from build123d import *
from OCP.BRepFilletAPI import BRepFilletAPI_MakeChamfer

# Parameters (mm, degrees)
BOSS_EXTRUDE1_START = -0.635
SKETCH3_R           = 9.525
SKETCH3_R_2         = 4.9657
BOSS_EXTRUDE1_DEPTH = 1.27
CHAMFER1_SIZE       = 0.127
CHAMFER1_SIZE2      = 0.073323484
FILLET1_R           = 0.381


with BuildPart() as part:
    # Sketch3 → Boss-Extrude1 (new body)
    with BuildSketch(Plane.XY.offset(BOSS_EXTRUDE1_START)):
        Circle(SKETCH3_R)
        Circle(SKETCH3_R_2, mode=Mode.SUBTRACT)
    extrude(amount=BOSS_EXTRUDE1_DEPTH)

    # Chamfer1: one chamfer whose edges measure the first distance from different faces: ONE call of the kernel's chamfer builder (chamfer() names one face for all edges)
    chamfer1_edges_1 = [part.edges().sort_by_distance(p)[0] for p in [
        (-9.525, 0, 0.635),
    ]]
    chamfer1_side_1 = [part.faces().sort_by_distance(p)[0] for p in [
        (-9.525, 0, 0),
    ]]
    chamfer1_edges_2 = [part.edges().sort_by_distance(p)[0] for p in [
        (-4.9657, 0, 0.635),
    ]]
    chamfer1_side_2 = [part.faces().sort_by_distance(p)[0] for p in [
        (-4.9657, 0, 0),
    ]]
    chamfer1 = BRepFilletAPI_MakeChamfer(part.part.solid().wrapped)
    for e in chamfer1_edges_1:
        chamfer1.Add(CHAMFER1_SIZE, CHAMFER1_SIZE2, e.wrapped, chamfer1_side_1[0].wrapped)  # the first distance lies on this face
    for e in chamfer1_edges_2:
        chamfer1.Add(CHAMFER1_SIZE, CHAMFER1_SIZE2, e.wrapped, chamfer1_side_2[0].wrapped)  # the first distance lies on this face
    add(Compound.cast(chamfer1.Shape()), mode=Mode.REPLACE)

    # Fillet1
    # the kernel refuses this fillet: 0.381 mm, written as the material it takes off along each edge
    with BuildSketch(Plane(origin=(0, 0, 0.635), x_dir=(1, 0, 0), z_dir=(0, -1, 0))) as fillet1_piece_1:
        with BuildLine():
            CenterArc((9.241019367, -0.381), FILLET1_R, 41.810314896, 48.189685104)
            Line((9.241019367, 0), (9.241019367, 0.00762))
            Line((9.241019367, 0.00762), (9.451676516, 0.00762))
            Line((9.451676516, 0.00762), (9.458275629, 0.00381))
            ThreePointArc((9.458275629, 0.00381), (9.494937371, -0.05969), (9.530679613, -0.12192))
            Line((9.530679613, -0.12192), (9.525, -0.127))
        make_face()
    revolve(axis=Axis((0, 0, 0.635), (0, 0, 1)), mode=Mode.SUBTRACT)
    with BuildSketch(Plane(origin=(0, 0, 0.635), x_dir=(1, 0, 0), z_dir=(0, -1, 0))) as fillet1_piece_2:
        with BuildLine():
            CenterArc((5.249680633, -0.381), FILLET1_R, 90, 48.189685104)
            Line((4.9657, -0.127), (4.960020387, -0.12192))
            ThreePointArc((4.960020387, -0.12192), (4.995762629, -0.05969), (5.032424371, 0.00381))
            Line((5.032424371, 0.00381), (5.039023484, 0.00762))
            Line((5.039023484, 0.00762), (5.249680633, 0.00762))
            Line((5.249680633, 0.00762), (5.249680633, 0))
        make_face()
    revolve(axis=Axis((0, 0, 0.635), (0, 0, 1)), mode=Mode.SUBTRACT)


solid = part.part
Part model, mm, in its own coordinate system. Coordinates: 2 decimals unless noted, no trailing zeros. Loops run counter-clockwise (first coordinate to the right, second up) from the corner with the lowest first, then second, coordinate; pieces in that order, holes last. Notation, with made-up numbers: M 66.25,64 L 108.25,64 A22 ccw 108.25,83 Z; hole C 83.25,11 d7. An arc over 180 degrees is marked long. Use a Markdown table: item, result. Add a question column.
Q1. Mould opens along Y. For faces 1 (the cylindrical face through (-7.559, -5.796, -0.072)), 2 (the flat face through (4, -4, -0.635)), 3 (the cylindrical face through (4.736, 1.492, -0.072)) say: +Y half, -Y half, draft (parallel to the pull), parting line (faces both ways), or undercut.
Q2. Probe L1, parallel to Y at x = 0, z = -0.1 (3 decimals); L2, parallel to Y at x = 3.25, z = 0; L3, parallel to X at y = -0.5, z = 0.55. List the from-to ranges inside material, lowest first.
Q3. Cut at A-A (x = 0). Write the cut outline in (y, z) (3 decimals).
Q4. Pin check, flat tip, straight feed: P1, Ø4, axis at x = 3, y = 3.5, coming from the -Z side (3 decimals). Stop position of the tip, or through.
Q5. Cut at C-C (z = 0). Write the cut outline in (x, y) (3 decimals), and give its area (3 significant figures).
Worked out:
| question | item | result |
|---|---|---|
| 1 | face 1 | parting line |
| 1 | face 2 | draft |
| 1 | face 3 | undercut |
| 2 | L1 | y = -9.525 to -4.966, 4.966 to 9.525 |
| 2 | L2 | y = -8.95 to -3.75, 3.75 to 8.95 |
| 2 | L3 | x = -9.47 to -4.98, 4.98 to 9.47 |
| 3 | outline | M -9.525,-0.635 L -4.966,-0.635 L -4.966,0.508 A0.381 ccw -5.25,0.635 L -9.241,0.635 A0.381 ccw -9.525,0.508 Z; M 4.966,-0.635 L 9.525,-0.635 L 9.525,0.508 A0.381 ccw 9.241,0.635 L 5.25,0.635 A0.381 ccw 4.966,0.508 Z |
| 4 | P1 | stops at z = -0.635 |
| 5 | outline | C 0,0 d19.05; hole C 0,0 d9.931 |
| 5 | area | 208 mm2 |
